Here's how the part is built. I have some questions about the finished solid (model axes, mm). A direction names the side the tool comes from. Round coordinates to 2 decimals unless told otherwise and drop trailing zeros. Loops run counter-clockwise (first coordinate to the right, second up) from the corner with the lowest first, then second, coordinate; pieces in that order, holes last. Notation, with made-up numbers: M 51,40 L 77,40 A18 ccw 77,51 Z; hole C 53,50.5 d8. An arc over 180 degrees is marked long. Write each question's results on one line, items separated by ' | '. Start each with the question number.
Autodesk Fusion 360 part; units mm, degrees
sketch "Sketch1" plane through (0, 0, 0) normal (0, 0, 1) x (1, 0, 0)
  line L0 (9, -9) -> (-9, -9)
  line L1 (-9, -9) -> (-9, 9)
  line L2 (-9, 9) -> (9, 9)
  line L3 (9, 9) -> (9, -9)
  line L4 (9, -9) -> (-9, 9) construction
  line L5 (-9, -9) -> (9, 9) construction
  dimension "d1" = 18
extrude "Extrude1" add sketch "Sketch1" along normal blind 17
sketch "Sketch2" plane through (0, 0, 17) normal (0, 0, 1) x (-1, 0, 0)
  line L0 (-9, -9) -> (9, -9)
  line L1 (9, -9) -> (9, 9)
  line L2 (9, 9) -> (-9, 9)
  line L3 (-9, 9) -> (-9, -9)
  line L4 (-7.34, 7.34) -> (7.34, 7.34)
  line L5 (7.34, 7.34) -> (7.34, -7.34)
  line L6 (7.34, -7.34) -> (-7.34, -7.34)
  line L7 (-7.34, -7.34) -> (-7.34, 7.34)
  line L8 (-7.34, 7.34) -> (7.34, -7.34) construction
  line L9 (7.34, 7.34) -> (-7.34, -7.34) construction
  dimension "d4" = 14.68
extrude "Extrude2" cut sketch "Sketch2" against normal blind 12 contours L4 L5 L6 L7
sketch "Sketch3" plane through (0, 0, 5) normal (0, 0, 1) x (-1, 0, 0)
  line L0 (-7.34, -7.34) -> (7.34, -7.34)
  line L1 (7.34, -7.34) -> (7.34, 7.34)
  line L2 (7.34, 7.34) -> (-7.34, 7.34)
  line L3 (-7.34, 7.34) -> (-7.34, -7.34)
  circle A0 centre (0, 0) radius 3.5
  dimension "d7" = 7
extrude "Extrude3" cut sketch "Sketch3" against normal blind 3 contours A0
sketch "Sketch4" plane through (0, 0, 2) normal (0, 0, 1) x (-1, 0, 0)
  circle A0 centre (0, 0) radius 3.5
  circle A1 centre (0, 0) radius 1.85
  dimension "d10" = 3.7
extrude "Extrude4" cut sketch "Sketch4" against normal blind 2 contours A1
sketch "Sketch5" plane through (0, -9, 0) normal (0, -1, 0) x (1, 0, 0)
  line L0 (-9, 0) -> (9, 0)
  line L1 (9, 0) -> (9, 17)
  line L2 (9, 17) -> (-9, 17)
  line L3 (-9, 17) -> (-9, 0)
  line L4 (-9, 17) -> (9, 17)
  line L5 (9, 17) -> (9, 15)
  line L6 (9, 15) -> (-9, 15)
  line L7 (-9, 15) -> (-9, 17)
  line L8 (-9, 5) -> (9, 5) construction
  dimension "d14" = 5
  dimension "d16" = 10
extrude "Extrude5" cut sketch "Sketch5" against normal blind 18 contours L1 L2 L3 L4 L5 L6 L7
sketch "Sketch6" plane through (0, -9, 0) normal (0, -1, 0) x (1, 0, 0)
  line L0 (9, 15) -> (-9, 15)
  line L1 (-9, 15) -> (-9, 0)
  line L2 (-9, 0) -> (9, 0)
  line L3 (9, 0) -> (9, 15)
  line L4 (-0.5, 15) -> (-0.5, 5.5)
  arc A0 (-0.5, 5.5) -> (0.5, 5.5) centre (0, 5.5) ccw
  line L5 (0.5, 5.5) -> (0.5, 15)
  line L6 (-9, 5) -> (9, 5) construction
  dimension "d19" = 5
  dimension "d20" = 1
extrude "Extrude6" cut sketch "Sketch6" against normal blind 1.66 contours L0 L4 A0 L5
Item 1: If we mould it in two halves opening along Y, with no side actions, what happens to faces 4 (the face through (-4, -7.34, 10)), 5 (the face through (0, 9, 7)), 6 (the face through (-2.1, 0.1, 0))? For each: released by +Y, released by -Y, zero draft, split by the parting line, or undercut.
Item 2: I'm going to push flat-ended pins straight in: pin 1 (6 mm diameter, centred on x = 0, y = 0, fed in from +Z); pin 2 (3.5 mm diameter, centred on x = -1.5, y = -1.5, fed in from +Z). Where does each tip first touch, or does it pass through?
Item 3: I need wall thicknesses on L1, parallel to X at y = 0, z = 3.15; L2, parallel to Y at x = 6.5, z = 14.25. Which ranges of each line are inside material? Lowest first, please.
Item 4: If we section it at A-A on y = 0: Please give me the cut outline in (x, z).
Item 5: If we section it at C-C on z = 1.25: Please give me the cut outline in (x, y).
Item 6: If we section it at B-B on x = -6.25: Please give me the cut outline in (y, z).
Item 7: If we section it at D-D on z = 6.5: Please give me the cut outline in (x, y), and give its area (3 significant figures).
Item 8: Which directions (+Z, -Z, +X, -X, +Y, -Y) give clear straight access to the entire face, cutting with the end or side of a thin tool? Please do faces 1 (the face through (0.5, -8, 10)), 2 (the face through (-2, 2, 2)), 3 (the face through (9, 0, 7)).
Numbers:
1) face 4: undercut | face 5: released by +Y | face 6: zero draft
2) pin 1: z = 2 | pin 2: z = 5
3) L1: -9 to -3.5, 3.5 to 9 | L2: -9 to -7.34, 7.34 to 9
4) outline: M -9,0 L -1.85,0 L -1.85,2 L -3.5,2 L -3.5,5 L -7.34,5 L -7.34,15 L -9,15 Z; M 1.85,0 L 9,0 L 9,15 L 7.34,15 L 7.34,5 L 3.5,5 L 3.5,2 L 1.85,2 Z
5) outline: M -9,-9 L 9,-9 L 9,9 L -9,9 Z; hole C 0,0 d3.7
6) outline: M -9,0 L 9,0 L 9,15 L 7.34,15 L 7.34,5 L -7.34,5 L -7.34,15 L -9,15 Z
7) outline: M -9,-9 L -0.5,-9 L -0.5,-7.34 L -7.34,-7.34 L -7.34,7.34 L 7.34,7.34 L 7.34,-7.34 L 0.5,-7.34 L 0.5,-9 L 9,-9 L 9,9 L -9,9 Z | area: 107 mm²
8) face 1: +Z, -Y | face 2: +Z | face 3: +Z, -Z, +X, +Y, -Y
